from build123d import *

# Parameters (mm, degrees)
SKETCH1_R           = 35
BOSS_EXTRUDE1_DEPTH = 7
SKETCH2_W           = 3.5
SKETCH2_H           = 10
SKETCH2_W_2         = 10
SKETCH2_H_2         = 3
SKETCH2_W_3         = 3
BOSS_EXTRUDE2_DEPTH = 6
SKETCH3_W           = 3.9
SKETCH3_H           = 22
BOSS_EXTRUDE3_DEPTH = 7
SKETCH4_R           = 1.05
CUT_EXTRUDE1_DEPTH  = 10
CIRPATTERN1_COUNT   = 3
SKETCH5_R           = 1.05
CUT_EXTRUDE2_DEPTH  = 75.18206665
CIRPATTERN2_COUNT   = 4
FILLET1_R           = 1


with BuildPart() as part:
    # Sketch1 → Boss-Extrude1 (new body)
    with BuildSketch(Plane(origin=(0, 0, 0), x_dir=(1, 0, 0), z_dir=(0, 1, 0))):
        with Locations(Location((0, 0, 0), (0, 0, 270))):
            Circle(SKETCH1_R)
    extrude(amount=BOSS_EXTRUDE1_DEPTH)

    # Sketch2 → Boss-Extrude2 (add)
    with BuildSketch(Plane(origin=(0, 7, 0), x_dir=(1, 0, 0), z_dir=(0, 1, 0))):
        with Locations((5.5, 27)):
            Rectangle(SKETCH2_W, SKETCH2_H)
        with Locations((-27, 5.25)):
            Rectangle(SKETCH2_W_2, SKETCH2_H_2)
        with Locations((-5.25, -27)):
            Rectangle(SKETCH2_W_3, SKETCH2_H)
        with Locations((27, -5.25)):
            Rectangle(SKETCH2_W_2, SKETCH2_H_2)
    extrude(amount=BOSS_EXTRUDE2_DEPTH)

    # Sketch3 → Boss-Extrude3 (add)
    with BuildSketch(Plane(origin=(0, 0, 0), x_dir=(1, 0, 0), z_dir=(0, 1, 0))):
        with Locations((3.05, 41)):
            Rectangle(SKETCH3_W, SKETCH3_H)
        with Locations((-3.05, 41)):
            Rectangle(SKETCH3_W, SKETCH3_H)
        Polygon((23.480762114, -19.330127019), (25.430762114, -15.952627944), (44.483320997, -26.952627944), (42.533320997, -30.330127019), align=None)
        Polygon((28.480762114, -10.669872981), (26.530762114, -14.047372056), (45.583320997, -25.047372056), (47.533320997, -21.669872981), align=None)
        Polygon((-28.480762114, -10.669872981), (-26.530762114, -14.047372056), (-45.583320997, -25.047372056), (-47.533320997, -21.669872981), align=None)
        Polygon((-23.480762114, -19.330127019), (-25.430762114, -15.952627944), (-44.483320997, -26.952627944), (-42.533320997, -30.330127019), align=None)
    extrude(amount=BOSS_EXTRUDE3_DEPTH)

    # Sketch4 → Cut-Extrude1 (cut)
    with BuildSketch(Plane(origin=(5, 0, 0), x_dir=(0, 0, -1), z_dir=(1, 0, 0))):
        with Locations((49.75, 3.5)):
            Circle(SKETCH4_R)
        with Locations((44.25, 3.5)):
            Circle(SKETCH4_R)
        with Locations((38.75, 3.5)):
            Circle(SKETCH4_R)
    cut_extrude1 = extrude(amount=-CUT_EXTRUDE1_DEPTH, mode=Mode.SUBTRACT)

    # CirPattern1: Cut-Extrude1 ×3 about axis
    cirpattern1_axis = Axis((0, 13.65, 0), (0, -1, 0))
    for i in range(1, CIRPATTERN1_COUNT):
        add(cut_extrude1.rotate(cirpattern1_axis, i * 360 / CIRPATTERN1_COUNT), mode=Mode.SUBTRACT)

    # Sketch5 → Cut-Extrude2 (cut, through all)
    with BuildSketch(Plane.ZY.offset(-3.75)):
        with Locations((-30, 10)):
            Circle(SKETCH5_R)
        with Locations((-24, 10)):
            Circle(SKETCH5_R)
    cut_extrude2 = extrude(amount=-CUT_EXTRUDE2_DEPTH, mode=Mode.SUBTRACT)

    # CirPattern2: Cut-Extrude2 ×4 about axis
    cirpattern2_axis = Axis((0, 13.65, 0), (0, -1, 0))
    for i in range(1, CIRPATTERN2_COUNT):
        add(cut_extrude2.rotate(cirpattern2_axis, i * 360 / CIRPATTERN2_COUNT), mode=Mode.SUBTRACT)

    # Fillet1
    fillet1_edges = [part.edges().sort_by_distance(p)[0] for p in [
        (5.5, 13, -22),
        (27.5, 3.5, 21.650635095),
        (43.508320997, 7, 28.641377482),
        (32.5, 3.5, 12.990381057),
        (46.558320997, 7, 23.358622518),
        (-32.5, 3.5, 12.990381057),
        (-46.558320997, 7, 23.358622518),
        (-27.5, 3.5, 21.650635095),
        (-43.508320997, 7, 28.641377482),
        (-3.75, 7, 27),
        (-5.25, 7, 22),
        (-6.75, 7, 27),
        (-5.25, 7, 32),
        (-5.25, 13, 22),
        (-5.25, 13, 32),
        (-22, 7, -5.25),
        (-27, 7, -6.75),
        (-32, 7, -5.25),
        (-27, 7, -3.75),
        (-22, 13, -5.25),
        (-32, 13, -5.25),
        (22, 7, 5.25),
        (27, 7, 6.75),
        (32, 7, 5.25),
        (27, 7, 3.75),
        (22, 13, 5.25),
        (32, 13, 5.25),
        (5, 3.5, -34.641016151),
        (3.05, 7, -52),
        (7.25, 7, -27),
        (5.5, 7, -32),
        (-5, 3.5, -34.641016151),
        (-3.05, 7, -52),
        (3.75, 7, -27),
        (5.5, 7, -22),
        (5.5, 13, -32),
    ]]
    fillet(fillet1_edges, radius=FILLET1_R)


solid = part.part
Verification items for the finished model (mm, model axes). A direction names the side the tool comes from. Give positions to 0.01 mm unless a question says otherwise; leave off trailing zeros. Order: outer loops, then holes, each group sorted by start corner. A loop starts at its lowest first (then second) coordinate and runs counter-clockwise, first axis right, second up. Notation, with made-up numbers: M 34.25,89.25 L 40.25,89.25 A16 cw 40.25,119.25 Z; hole C 31.25,51.5 d5. An arc over 180 degrees is marked long. Use one line per item in the form item = value. Start each with the question number.
Q1. Section check A-A (z = -49.75). Enter the section's corners in (x, y).
Q2. Mould release check, pull along X, two halves, no side actions. Record for faces 6 (the flat face through (32, 10, 5)), 7 (the flat face through (27, 13, 5)), 8 (the cylindrical face through (-36.69, 4.54, 24.67)): +X half, -X half, draft (parallel to the pull), parting line (faces both ways), or undercut.
Q3. Access from +Z, -Z, +X, -X, +Y, -Y to the whole of each face (thin tool, end or side, straight path). Record for faces 1 (the flat face through (-5, 5, -44)), 2 (the flat face through (-1.1, 3, -43)), 3 (the flat face through (38.111, 2.673, 20.733)), 4 (the flat face through (5, 10, -32)), 5 (the flat face through (40.487, 5.007, 17.602)).
Q4. Go/stop test with flat-tipped pins: pin 1 Ø5.5 at (y, z) = (3, -45) entering from -X; pin 2 Ø6 at (y, z) = (10.5, -25.5) entering from +X; pin 3 Ø1.3 at (x, y) = (24, 10) entering from +Z; pin 4 Ø0.9 at (y, z) = (9.5, -5) entering from -X. Record where each tip stops, or that it passes through.
Q5. Scan lines: line 1 along X through (y, z) = (6.5, -45.5); line 2 along Y through (x, z) = (-3.6, -49.75); line 3 along Y through (x, z) = (6.5, -30). Record each from-to range of solid material in increasing order. Write a range as [from, to].
Q6. Section check C-C (y = 3.5). Count the separate pieces of the cut face and the enclosed holes in it, then the cut area to 3 significant figures.
Q7. Section check B-B (z = -5). Enter the section's corners in (x, y), then the cut area to 3 significant figures.
Evaluation:
q1.outline = M -5,0 L -1.1,0 L -1.1,2.45 L -5,2.45 Z; M -5,4.55 L -1.1,4.55 L -1.1,7 L -5,7 Z; M 1.1,0 L 5,0 L 5,2.45 L 1.1,2.45 Z; M 1.1,4.55 L 5,4.55 L 5,7 L 1.1,7 Z
q2.face_6 = +X half
q2.face_7 = draft
q2.face_8 = undercut
q3.face_1 = -Z, -X, +Y, -Y
q3.face_2 = -Z, +Y, -Y
q3.face_3 = +Y, -Y
q3.face_4 = -Z, +X, -X, +Y
q3.face_5 = +X, +Y, -Y
q4.pin_1 = -5
q4.pin_2 = 7.38
q4.pin_3 = through
q4.pin_4 = -32
q5.line_1 = [-5, -1.1], [1.1, 5]
q5.line_2 = [0, 2.45], [4.55, 7]
q5.line_3 = [0, 8.95], [11.05, 13]
q6.separate_pieces = 19
q6.enclosed_holes = 0
q6.area = 4,100 mm2
q7.outline = M -34.64,0 L 34.64,0 L 34.64,7 L -21,7 A1 cw -22,8 L -22,12 A1 ccw -23,13 L -31,13 A1 ccw -32,12 L -32,8 A1 cw -33,7 L -34.64,7 Z; hole C -30,10 d2.1; hole C -24,10 d2.1
q7.area = 538 mm2
